Autodesk Inventor part; units mm, degrees
ref_plane "YZ Plane" through (0, 0, 0) normal (1, 0, 0) x (0, 1, 0)
ref_plane "XZ Plane" through (0, 0, 0) normal (0, 1, 0) x (-1, 0, 0)
ref_plane "XY Plane" through (0, 0, 0) normal (0, 0, 1) x (1, 0, 0)
sketch "Эскиз1" plane through (0, 0, 0) normal (0, 0, 1) x (1, 0, 0)
  line L0 (0, 0) -> (0, 15) construction
  line L1 (0, 0) -> (-22, 0) construction
  circle A0 centre (0, 0) radius 2.15
  circle A1 centre (0, 0) radius 8
  circle A2 centre (0, 0) radius 6
  circle A3 centre (0, 0) radius 5
  dimension "d0" = 4.3
  dimension "d1" = 16
  dimension "d2" = 12
  dimension "d3" = 10
extrude "Выдавливание1" add sketch "Эскиз1" along normal blind 3.8 contours A1 | A2 | A3
extrude "Выдавливание2" add sketch "Эскиз1" against normal blind 9 contours A1 | A2
extrude "Выдавливание3" cut sketch "Эскиз1" against normal blind 6 contours A1
extrude "Выдавливание4" add sketch "Эскиз1" against normal blind 2.2 contours A3
chamfer "Фаска1" distance 2.85 distance2 1 1 edges at (-2.15, 0, -2.2) measured on face at (4.0016, -0.3989, -2.2)
sketch "Эскиз2" plane through (0, 0, -9) normal (0, 0, -1) x (-1, 0, 0)
  circle A0 centre (0, 0) radius 5
  circle A1 centre (0, 0) radius 3.25
  dimension "d15" = 10
  dimension "d16" = 6.5
extrude "Выдавливание5" add sketch "Эскиз2" along normal blind 0.5 and the other way blind 2
chamfer "Фаска2" distance 0.8 angle 45 1 edges at (3.25, 0, -9.5)
fillet "Сопряжение1" radius 0.1 1 edges at (5, 0, -9.5)
chamfer "Фаска3" distance 0.8 angle 45 1 edges at (-2.15, 0, 3.8)
chamfer "Фаска4" distance 0.3 angle 45 4 edges at (-8, 0, 3.8) (-8, 0, 0) (-8, 0, -6) (-8, 0, -9)
properties part number "втулка фитинг"
Work out the finished part from the listing and answer in its coordinate system (mm). A direction names the side the tool comes from. Round coordinates to 2 decimals unless told otherwise and drop trailing zeros. Loops run counter-clockwise (first coordinate to the right, second up) from the corner with the lowest first, then second, coordinate; pieces in that order, holes last. Notation, with made-up numbers: (45.25, 78) - (70.25, 78) arc R22 cw to (70.25, 106) - close; hole circle Ø7 at (73, 73.5). An arc over 180 degrees is marked (long way). One line per item, written item: value.
Q1. Each of these flat-tipped pins is pushed along its axis until it touches: pin 1 Ø5 at (x, y) = (2, 1) entering from -Z; pin 2 Ø1 at (x, y) = (5, 5) entering from -Z; pin 3 Ø1.5 at (y, z) = (1.5, 0.5) entering from +X; pin 4 Ø2 at (y, z) = (-6, -7.5) entering from +X (3 decimals). Where does it stop, or does it pass through?
Check values:
pin 1: z = -9.5
pin 2: z = -9
pin 3: x = 7.96
pin 4: x = 6.245
Q2. For faces 5 (the flat face through (2, -5, -9)), 6 (the conical face through (-0.5, 2.27, -1.26)), 7 (the cylindrical face through (-2.15, 0.09, 0.93)), determine the directions among +Z, -Z, +X, -X, +Y, -Y from which every point of the face is accessible in a straight line to the end or side of a thin tool.
Check values:
face 5: -Z
face 6: none
face 7: +Z, -Z
Q3. The mould has two halves that part along X. Classify faces 1 (the cylindrical face through (0.705, -3.173, -7.862)), 2 (the cylindrical face through (-1.08, -4.88, -4.57)), 3 (the flat face through (5, -4, -6)), 4 (the cylindrical face through (-6, 0, -3)): +X half, -X half, draft (parallel to the pull), parting line (faces both ways), or undercut.
Check values:
face 1: undercut
face 2: undercut
face 3: draft
face 4: parting line
Q4. Straight lines are drawn through the part: probe 1 along Z at (x, y) = (1.75, -6.5); probe 2 along Y at (x, z) = (0, -7.5); probe 3 along Y at (x, z) = (0, -4.95). For each, find the intervals that lie inside material, in ascending order.
Check values:
probe 1: -9 to -6, 0 to 3.8
probe 2: -8 to -3.25, 3.25 to 8
probe 3: -6 to -5, 5 to 6
Q5. Find section A-A on z = -2.5. Give the vertices of the cut face in (x, y).
Check values:
outline: circle Ø12 at (0, 0); hole circle Ø10 at (0, 0)
